from build123d import *

# Parameters (mm, degrees)
F1_DEPTH = 2.286


with BuildPart() as f1:
    # F0 (on Top) → F1 (new body)
    with BuildSketch(Plane.XY):
        with BuildLine():
            ThreePointArc((0, 3.81), (1.115923, 1.115923), (3.81, 0))
            Line((3.81, 0), (10.16, 0))
            Line((10.16, 0), (10.16, 7.62))
            Line((10.16, 7.62), (3.81, 7.62))
            ThreePointArc((3.81, 7.62), (1.115923, 6.504077), (0, 3.81))
        make_face()
        with BuildLine():
            ThreePointArc((5.08, 3.81), (3.81, 2.54), (2.54, 3.81))
            ThreePointArc((2.54, 3.81), (3.81, 5.08), (5.08, 3.81))
        make_face(mode=Mode.SUBTRACT)
    extrude(amount=F1_DEPTH)


solid = f1.part
Geometry: final body of the model. Coordinates: model frame, mm. Give positions to 0.01 mm unless a question says otherwise; leave off trailing zeros. Write each loop counter-clockwise with the first axis right and the second up, starting at its lowest first coordinate (ties: lowest second). Pieces come first, ordered by that corner, then holes. Notation, with made-up numbers: M 87,85 L 120,85 A12 cw 120,95 Z; hole C 16.25,84.25 d3. An arc over 180 degrees is marked long. Answer in a Markdown table with one row per item. Add a question column.
(1) First-contact query: pin 1 (3.5 mm diameter, centred on x = 3.81, y = 3.81, fed in from -Z). Flat tip, straight axial feed; report the tip coordinate or a pass-through.
(2) Section A-A on y = 3.25. Return loops of the section in (x, z), and give its area (3 significant figures).
(3) Section D-D on x = 1.25. Return loops of the section in (y, z).
(4) Mould query, pull axis X, two halves, no side actions, for faces 1 (the flat face through (10.16, 4, 1)), 2 (the flat face through (7, 0, 1)), 3 (the cylindrical face through (3.224, 2.683, 1.127)). Classes: +X half, -X half, draft (parallel to the pull), parting line (faces both ways), or undercut.
(5) Section C-C on y = 2.25. Return loops of the section in (x, z).
(6) Section B-B on z = 0.5. Return loops of the section in (x, y).
(7) Ray query, line 1 (Y direction, x = 3.81, z = 1.2); line 2 (Y direction, x = 3.5, z = 0.65); line 3 (Y direction, x = 1, z = 2.15). Return the intervals inside material, ascending.
Result set:
| question | item | result |
|---|---|---|
| 1 | pin 1 | stops at z = 0 |
| 2 | outline | M 0.04,0 L 2.67,0 L 2.67,2.29 L 0.04,2.29 Z; M 4.95,0 L 10.16,0 L 10.16,2.29 L 4.95,2.29 Z |
| 2 | area | 17.9 mm^2 |
| 3 | outline | M 0.99,0 L 6.63,0 L 6.63,2.29 L 0.99,2.29 Z |
| 4 | face 1 | +X half |
| 4 | face 2 | draft |
| 4 | face 3 | undercut |
| 5 | outline | M 0.33,0 L 10.16,0 L 10.16,2.29 L 0.33,2.29 Z |
| 6 | outline | M 0,3.81 A3.81 ccw 3.81,0 L 10.16,0 L 10.16,7.62 L 3.81,7.62 A3.81 ccw Z; hole C 3.81,3.81 d2.54 |
| 7 | line 1 | y = 0 to 2.54, 5.08 to 7.62 |
| 7 | line 2 | y = 0.01 to 2.58, 5.04 to 7.61 |
| 7 | line 3 | y = 1.24 to 6.38 |
